Part model, mm, in its own coordinate system. Give positions to 0.01 mm unless a question says otherwise; leave off trailing zeros. Write each loop counter-clockwise with the first axis right and the second up, starting at its lowest first coordinate (ties: lowest second). Pieces come first, ordered by that corner, then holes. Notation, with made-up numbers: (34, 59) - (90, 59) arc R9 cw to (90, 63) - close; hole circle Ø7 at (56.25, -27). An arc over 180 degrees is marked (long way). Answer as a JSON object with one key per item and string values. Group by question number.
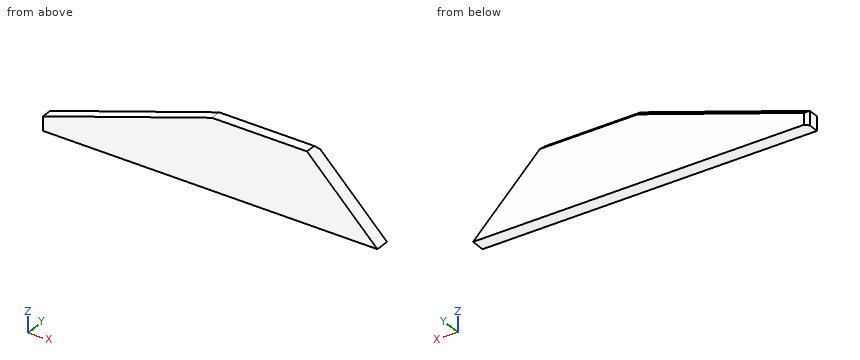
```python
from build123d import *

# Parameters (mm, degrees)
F1_DEPTH = 20
F2_SIZE  = 5
F3_SIZE  = 99.99999


# Not quite as in the source:
# - a fillet or chamfer is up to 0.001 mm smaller than in the source, because OpenCascade refuses the exact size


with BuildPart() as f1:
    # F0 (on Front) → F1 (new body)
    with BuildSketch(Plane.XZ):
        Polygon((-227.9723286629, -18.1198753417), (247.0276713371, -18.1198753417), (247.0276713371, 81.8801246583), (12.0276713371, 81.8801246583), (-227.9723286629, 1.8801246583), align=None)
    extrude(amount=F1_DEPTH)

    # F2
    f2_edges = [f1.edges().sort_by_distance(p)[0] for p in [
        (129.527671, 0, 81.880125),
        (-107.972329, 0, 41.880125),
        (-227.972329, 0, -8.119875),
    ]]
    chamfer(f2_edges, length=F2_SIZE)

    # F3 (size 100 in the source; OpenCascade refuses exactly that, so slightly less here)
    f3_edges = [f1.edges().sort_by_distance(p)[0] for p in [
        (247.027671, -12.5, 81.880125),
    ]]
    chamfer(f3_edges, length=F3_SIZE)


solid = f1.part
```
1) Band-saw the part on C-C (z = 66.5). List the corners of the cut face in (x, y).
2) Band-saw the part on D-D (x = 213). List the corners of the cut face in (y, z), plus the area to 3 significant figures.
3) Band-saw the part on B-B (x = -92.5). List the corners of the cut face in (y, z).
4) Drop flat-ended pins along their axis: P1, Ø4, axis at y = -14.5, z = 30.5, coming from the +X side; P2, Ø10, axis at y = -9, z = 46, coming from the +X side; P3, Ø4, axis at x = -71.5, y = -6, coming from the +Z side. Give the stop position or say it passes through.
5) Probe line 1 (X direction, y = -19, z = -5); line 2 (X direction, y = -3, z = -12); line 3 (Z direction, x = -125.5, y = -12.5). List the from-to ranges inside material, lowest first.
Verdict:
{
 "1": {"outline": "(-34.11, -20) - (162.41, -20) - (162.41, 0) - (-18.3, 0) - (-34.11, -5) - close"},
 "2": {"outline": "(-20, -18.12) - (0, -18.12) - (0, 15.91) - (-20, 15.91) - close", "area": "681 mm2"},
 "3": {"outline": "(-20, -18.12) - (0, -18.12) - (0, 41.77) - (-5, 47.04) - (-20, 47.04) - close"},
 "4": {"P1": "x = 200.41", "P2": "x = 187.91", "P3": "z = 54.7"},
 "5": {"line 1": "-227.97 to 233.91", "line 2": "-225.97 to 240.91", "line 3": "-18.12 to 36.04"}
}
